Check sheet for the modelled part. Datum: model origin and axes. Units: mm. A direction names the side the tool comes from. Round coordinates to 2 decimals unless told otherwise and drop trailing zeros. Loops run counter-clockwise (first coordinate to the right, second up) from the corner with the lowest first, then second, coordinate; pieces in that order, holes last. Notation, with made-up numbers: M 29,18.5 L 67,18.5 A32 cw 67,57.5 Z; hole C 8.5,-25 d6. An arc over 180 degrees is marked long. One line per question, with ' | ' between items. Start each with the question number.
(1) Section check A-A (z = -105). Record the boundary of the cut face in (x, y), and give its area (3 significant figures).
(2) Tool access check on faces 1 (the face through (5, 8, -67)), 2 (the face through (5, 0, -27)), 3 (the face through (5, 20, -108)), 4 (the face through (5, -3, -100)), 5 (the face through (5, 15, -106)). Record the directions out of +Z, -Z, +X, -X, +Y, -Y that give a thin tool (end or side, any length) a straight path to the whole face; none if there is none.
(3) Thickness scan on probe 1 along Z at (x, y) = (8.25, -5); probe 2 along Y at (x, z) = (3, -55); probe 3 along Y at (x, z) = (5.25, -34). Record the ranges inside material, lowest first. Write a range as [from, to].
(4) Section check C-C (y = 12.5). Record the boundary of the cut face in (x, z), and give its area (3 significant figures).
(5) Section check B-B (x = 4). Count the separate pieces of the cut face and the enclosed holes in it, and give its area (3 significant figures).
(6) Draft check along Z on faces 6 (the face through (5, 6, -87)), 7 (the face through (5, 8, -110)), 8 (the face through (4.93, -0.6, -60.57)), 9 (the face through (5, 2, -1)). Enter one of: +Z half, -Z half, draft (parallel to the pull), parting line (faces both ways), or undercut.
(7) Section check D-D (z = -54). Record the boundary of the cut face in (x, y), and give its area (3 significant figures).
(8) Go/stop test with flat-tipped pins: P1, Ø6, axis at x = 3, z = -50, coming from the -Y side; P2, Ø6, axis at x = 6, z = -17.5, coming from the -Y side; P3, Ø4, axis at x = 6, y = -0.5, coming from the +Z side; P4, Ø4, axis at y = 13.5, z = -63.5, coming from the +X side. Record where each tip stops, or that it passes through.
Autodesk Inventor part; units mm, degrees
ref_plane "YZ Plane" through (0, 0, 0) normal (1, 0, 0) x (0, 1, 0)
ref_plane "XZ Plane" through (0, 0, 0) normal (0, 1, 0) x (-1, 0, 0)
ref_plane "XY Plane" through (0, 0, 0) normal (0, 0, 1) x (1, 0, 0)
sketch "Эскиз1" plane through (0, 0, 0) normal (1, 0, 0) x (0, 1, 0)
  line L0 (0, 0) -> (10, 0)
  line L1 (10, 0) -> (10, -110)
  line L2 (10, -110) -> (0, -110)
  line L3 (0, -110) -> (0, 0)
  line L4 (10, -110) -> (20, -110)
  line L5 (20, -110) -> (20, -106)
  line L6 (20, -106) -> (10, -106)
  line L7 (10, -106) -> (10, -110)
  dimension "d0" = 110
  dimension "d1" = 10
  dimension "d2" = 4
  dimension "d3" = 10
extrude "Выдавливание1" add sketch "Эскиз1" along normal blind 10
sketch "Эскиз2" plane through (0, 10, 0) normal (0, 1, 0) x (1, 0, 0)
  line L0 (0, 106) -> (10, 106)
  line L1 (5, 106) -> (5, 0)
  line L2 (0, 0) -> (10, 0)
  line L3 (7, 82) -> (3, 82)
  line L4 (3, 82) -> (3, 92)
  line L5 (3, 92) -> (7, 92)
  line L6 (7, 92) -> (7, 82)
  line L7 (7, 57) -> (3, 57)
  line L8 (3, 57) -> (3, 67)
  line L9 (3, 67) -> (7, 67)
  line L10 (7, 67) -> (7, 57)
  line L11 (7, 32) -> (3, 32)
  line L12 (3, 32) -> (3, 42)
  line L13 (3, 42) -> (7, 42)
  line L14 (7, 42) -> (7, 32)
  line L15 (7, 7) -> (3, 7)
  line L16 (3, 7) -> (3, 17)
  line L17 (3, 17) -> (7, 17)
  line L18 (7, 17) -> (7, 7)
  dimension "d6" = 10
  dimension "d7" = 10
  dimension "d8" = 10
  dimension "d9" = 10
  dimension "d10" = 4
  dimension "d11" = 4
  dimension "d12" = 4
  dimension "d13" = 14
  dimension "d14" = 15
  dimension "d15" = 15
  dimension "d16" = 15
extrude "Выдавливание2" cut sketch "Эскиз2" against normal blind 4
sketch "Эскиз3" plane through (10, 0, 0) normal (1, 0, 0) x (0, 0, -1)
  line L0 (106, 10) -> (0, 10)
  line L1 (0, 10) -> (-10, 10)
  line L2 (-10, 10) -> (-10, 0)
  line L3 (-10, 0) -> (0, 0)
  line L4 (0, 0) -> (0, 10)
  circle A0 centre (-5, 5) radius 5
  point P0 (-5, 10)
  point P1 (0, 5)
  dimension "d19" = 10
extrude "Выдавливание3" add sketch "Эскиз3" against normal blind 10 contours L4 A0 L1
fillet "Сопряжение1" radius 5 1 edges at (5, 0, 0)
sketch "Эскиз4" plane through (10, 0, 0) normal (1, 0, 0) x (0, 0, -1)
  line L0 (110, 0) -> (100, 0)
  line L1 (100, 0) -> (100, -5)
  line L2 (100, -5) -> (110, -5)
  line L3 (110, -5) -> (110, 0)
  circle A0 centre (105, -5) radius 5
  circle A1 centre (105, -5) radius 2
  line L4 (5, 0) -> (110, 0)
  line L5 (60, 0) -> (50, 0)
  line L6 (50, 0) -> (50, -5)
  line L7 (50, -5) -> (60, -5)
  line L8 (60, -5) -> (60, 0)
  circle A2 centre (55, -5) radius 5
  circle A3 centre (55, -5) radius 2
  point P0 (0, 0)
  dimension "d23" = 10
  dimension "d24" = 5
  dimension "d25" = 4
  dimension "d26" = 10
  dimension "d27" = 5
  dimension "d28" = 4
  dimension "d29" = 40
extrude "Выдавливание4" add sketch "Эскиз4" against normal blind 10 contours L3 A0 L0 | L8 A2 L4 | A0 L1 L0 | A0 L2 A1 | A0 L2 A1 | A2 L6 L4 | A2 L7 A3 | A2 L7 A3
fillet "Сопряжение2" radius 2 3 edges at (5, 0, -100) (5, 0, -50) (5, 0, -60)
properties part number "держак середины пушки"
The answers:
1) outline: M 0,-10 L 10,-10 L 10,-7 L 0,-7 Z; M 0,-3 L 10,-3 L 10,10 L 0,10 Z | area: 160 mm²
2) face 1: +Y | face 2: +Z, +X, -X, -Y | face 3: +Z, -Z, +X, -X, +Y | face 4: +X, -X, -Y | face 5: +Z, +X, -X, +Y
3) probe 1: [-110, -107], [-103, -100], [-60, -57], [-53, -50] | probe 2: [-10, -7], [-3, 10] | probe 3: [0, 6]
4) outline: M 0,-110 L 10,-110 L 10,-106 L 0,-106 Z | area: 40.0 mm²
5) separate pieces: 1 | enclosed holes: 2 | area: 1,140 mm²
6) face 6: undercut | face 7: -Z half | face 8: undercut | face 9: +Z half
7) outline: M 0,-9.9 L 10,-9.9 L 10,-6.73 L 0,-6.73 Z; M 0,-3.27 L 10,-3.27 L 10,10 L 0,10 Z | area: 164 mm²
8) P1: y = -9.58 | P2: y = 0 | P3: z = -1.43 | P4: through
